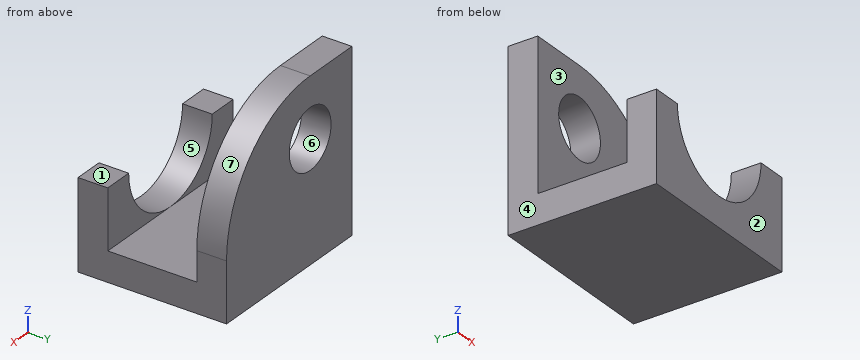
```python
from build123d import *

# Parameters (mm, degrees)
F0_W     = 152.4
F0_H     = 152.4
F1_DEPTH = 63.5
F3_DEPTH = 152.401
F5_DEPTH = 25.4
F6_R     = 25.4
F7_DEPTH = 25.4


with BuildPart() as f1:
    # F0 (on Front) → F1 (new body, symmetric)
    with BuildSketch(Plane.XZ):
        Rectangle(F0_W, F0_H)
    extrude(amount=F1_DEPTH, both=True)

    # F2 (on face) → F3 (cut, through all)
    with BuildSketch(Plane.YZ.offset(76.2)):
        Polygon((38.1, 76.2), (-38.1, 76.2), (-38.1, -50.8), (0, -50.8), (38.1, -50.8), align=None)
    extrude(amount=-F3_DEPTH, mode=Mode.SUBTRACT)

    # F4 (on face) → F5 (cut, through all)
    with BuildSketch(Plane.XZ.offset(63.5)):
        with BuildLine():
            Line((76.2, 0), (76.2, 76.2))
            Line((76.2, 76.2), (-76.2, 76.2))
            Line((-76.2, 76.2), (-76.2, 0))
            Line((-76.2, 0), (-50.8, 0))
            ThreePointArc((-50.8, 0), (0, 50.8), (50.8, 0))
            Line((50.8, 0), (76.2, 0))
        make_face()
        with BuildLine():
            Line((-50.8, 0), (50.8, 0))
            ThreePointArc((50.8, 0), (0, 50.8), (-50.8, 0))
        make_face()
        with BuildLine():
            ThreePointArc((-50.8, 0), (0, -50.8), (50.8, 0))
            Line((50.8, 0), (-50.8, 0))
        make_face()
    extrude(amount=-F5_DEPTH, mode=Mode.SUBTRACT)

    # F6 (on face) → F7 (cut, through all)
    with BuildSketch(Plane(origin=(0, 63.5, 0), x_dir=(-1, 0, 0), z_dir=(0, 1, 0))):
        with BuildLine():
            Line((25.3999998624, 76.2), (-76.2, 76.2))
            Line((-76.2, 76.2), (-76.2, -25.4))
            ThreePointArc((-76.2, -25.4), (-46.4420490172, 46.4420489199), (25.3999998624, 76.2))
        make_face()
        with Locations((25.4, 25.4)):
            Circle(F6_R)
    extrude(amount=-F7_DEPTH, mode=Mode.SUBTRACT)


solid = f1.part
```
Design review of the part built by this model. Coordinates are the model's own, in mm. Face numbers are marked on the shaded views. A direction names the side the tool comes from. Give positions to 0.01 mm unless a question says otherwise; leave off trailing zeros. Loops run counter-clockwise (first coordinate to the right, second up) from the corner with the lowest first, then second, coordinate; pieces in that order, holes last. Notation, with made-up numbers: (-33.75, -21) -> (10.25, -21) arc R6 ccw to (10.25, -17) -> close; hole circle Ø1 at (75.25, 9). An arc over 180 degrees is marked (long way). One line per item, written item: value.
Q1. For L1, parallel to Y at x = -63, z = -12.5; L2, parallel to Z at x = -25, y = 51; L3, parallel to Y at x = 25, z = -38, list the stretches that pass through material, from the lowest coordinate up.
Numbers:
L1: y = -63.5 to -38.1, 38.1 to 63.5
L2: z = -76.2 to 0, 50.8 to 76.2
L3: y = 38.1 to 63.5
Q2. Draft analysis for pull direction X (two halves, no side actions). For the marked faces 4, 5, 6 and 7, state which applies: pulls with the +X half, pulls with the -X half, needs draft (parallel to the pull), parting line crosses it, or undercut.
Numbers:
face 4: pulls with the -X half
face 5: undercut
face 6: undercut
face 7: pulls with the +X half
Q3. We need section A-A on z = -17. Give the boundary of the cut face in (x, y), and give its area (3 significant figures).
Numbers:
outline: (-76.2, -63.5) -> (-47.87, -63.5) -> (-47.87, -38.1) -> (-76.2, -38.1) -> close; (-76.2, 38.1) -> (75.85, 38.1) -> (75.85, 63.5) -> (-76.2, 63.5) -> close; (47.87, -63.5) -> (76.2, -63.5) -> (76.2, -38.1) -> (47.87, -38.1) -> close
area: 5,300 mm^2
Q4. We need section D-D on y = -52.5. Give the boundary of the cut face in (x, z).
Numbers:
outline: (-76.2, -76.2) -> (76.2, -76.2) -> (76.2, 0) -> (50.8, 0) arc R50.8 cw to (-50.8, 0) -> (-76.2, 0) -> close
Q5. For pin 1 Ø6 at (x, y) = (6.5, 7) entering from +Z; pin 2 Ø8 at (x, z) = (57.5, 1) entering from -Y; pin 3 Ø20.5 at (x, y) = (61.5, -56.5) entering from +Z, all flat-tipped, find the tip position at first contact; note any pin that passes through.
Numbers:
pin 1: stops at z = -50.8
pin 2: stops at y = -63.5
pin 3: stops at z = 0
Q6. Machinability: for the marked faces 1, 2 and 3, which of the approach directions +Z, -Z, +X, -X, +Y, -Y give a long, thin tool a straight path to every point of the face, cutting with its end or side? Answer none if there is none.
Numbers:
face 1: +Z, +X, -X, -Y
face 2: +Z, -Z, +X, -X, -Y
face 3: +Z, +X, -X
Q7. We need section C-C on x = -8.5. Give the boundary of the cut face in (y, z), and give its area (3 significant figures).
Numbers:
outline: (-63.5, -76.2) -> (63.5, -76.2) -> (63.5, 6.44) -> (38.1, 6.44) -> (38.1, -50.8) -> (-38.1, -50.8) -> (-38.1, -50.08) -> (-63.5, -50.08) -> close; (38.1, 44.36) -> (63.5, 44.36) -> (63.5, 74.78) -> (38.1, 74.78) -> close
area: 5,470 mm^2
Q8. We need section B-B on z = 18.5. Give the boundary of the cut face in (x, y), and give its area (3 significant figures).
Numbers:
outline: (-76.2, 38.1) -> (-49.84, 38.1) -> (-49.84, 63.5) -> (-76.2, 63.5) -> close; (-0.96, 38.1) -> (66.23, 38.1) -> (66.23, 63.5) -> (-0.96, 63.5) -> close
area: 2,380 mm^2
